from build123d import *

# Parameters (mm, degrees)
F0_W     = 294.005
F0_H     = 558.8
F1_DEPTH = 12.7
F3_D     = 4.4
F4_R     = 9.525
F6_DEPTH = 12.701


with BuildPart() as f1:
    # F0 (on Front) → F1 (new body)
    with BuildSketch(Plane.XZ):
        Rectangle(F0_W, F0_H)
    extrude(amount=F1_DEPTH)

    # F3 (through all)
    with Locations(Plane.XZ.offset(12.7)):
        with Locations((-137.4775, 269.875), (-105.7275, 269.875), (105.7275, 269.875), (137.4775, 269.875), (105.7275, -238.125), (137.4775, -238.125), (137.4775, -269.875), (105.7275, -269.875), (-105.7275, -269.875), (-137.4775, -269.875), (-137.4775, -238.125), (-105.7275, -238.125)):
            Hole(F3_D / 2)

    # F4
    f4_edges = [f1.edges().sort_by_distance(p)[0] for p in [
        (147.0025, -6.35, 279.4),
        (147.0025, -6.35, -279.4),
        (-147.0025, -6.35, -279.4),
        (-147.0025, -6.35, 279.4),
    ]]
    fillet(f4_edges, radius=F4_R)

    # F5 (on face) → F6 (cut, through all)
    with BuildSketch(Plane.XZ.offset(12.7)):
        with BuildLine():
            Line((88.9, 127), (-88.9, 127))
            ThreePointArc((-88.9, 127), (-106.8605122421, 119.5605122421), (-114.3, 101.6))
            Line((-114.3, 101.6), (-114.3, -203.2))
            ThreePointArc((-114.3, -203.2), (-106.8605122421, -221.1605122421), (-88.9, -228.6))
            Line((-88.9, -228.6), (88.9, -228.6))
            ThreePointArc((88.9, -228.6), (106.8605122421, -221.1605122421), (114.3, -203.2))
            Line((114.3, -203.2), (114.3, 101.6))
            ThreePointArc((114.3, 101.6), (106.8605122421, 119.5605122421), (88.9, 127))
        make_face()
    extrude(amount=-F6_DEPTH, mode=Mode.SUBTRACT)


solid = f1.part
Design review of the part built by this model. Coordinates are the model's own, in mm. A direction names the side the tool comes from. Give positions to 0.01 mm unless a question says otherwise; leave off trailing zeros. Order: outer loops, then holes, each group sorted by start corner. A loop starts at its lowest first (then second) coordinate and runs counter-clockwise, first axis right, second up. Notation, with made-up numbers: (71.5, 30.25) - (97.5, 30.25) arc R18 cw to (97.5, 40.25) - close; hole circle Ø5 at (-37.5, 44.25). An arc over 180 degrees is marked (long way). Use CSV: the item, a comma, the result in double quotes. Start each with the question number.
Q1. Draft analysis for pull direction Z (two halves, no side actions). For faces 1 (the face through (147.002, -6, -4)), 2 (the face through (144.14, -6.44, 276.68)), 3 (the face through (-107.06, -6.44, -220.96)), state which applies: pulls with the +Z half, pulls with the -Z half, needs draft (parallel to the pull), parting line crosses it, or undercut.
Q2. For P1, Ø7, axis at x = 105.73, z = -238.12, coming from the +Y side, flat-tipped, find the tip position at first contact; note if it passes through.
Q3. Machinability: for faces 4 (the face through (144.14, -6.44, -276.68)), 5 (the face through (107.06, -6.44, 119.36)), which of the approach directions +Z, -Z, +X, -X, +Y, -Y give a long, thin tool a straight path to every point of the face, cutting with its end or side? Answer none if there is none.
Q4. Take a section at B-B (x = -39.5). State the section outline as (y, z) points, and give its area (3 significant figures).
Q5. For line 1 (Z direction, x = -14, y = -7); line 2 (X direction, y = -7.75, z = 95); line 3 (Z direction, x = 99, y = -3.75), list the stretches that pass through material, from the lowest coordinate up.
Q6. Take a section at A-A (z = -44). State the section outline as (x, y) points, and give its area (3 significant figures).
Q7. Take a section at C-C (y = -7.25). Count the separate pieces of the cut face and the enclosed holes in it, and give its area (3 significant figures).
Calculated:
1,face 1,"needs draft"
1,face 2,"pulls with the +Z half"
1,face 3,"undercut"
2,P1,"stops at y = 0"
3,face 4,"-Z, +X, +Y, -Y"
3,face 5,"+Y, -Y"
4,outline,"(-12.7, -279.4) - (0, -279.4) - (0, -228.6) - (-12.7, -228.6) - close; (-12.7, 127) - (0, 127) - (0, 279.4) - (-12.7, 279.4) - close"
4,area,"2,580 mm²"
5,line 1,"z = -279.4 to -228.6, 127 to 279.4"
5,line 2,"x = -147 to -114.3, 114.3 to 147"
5,line 3,"z = -279.4 to -226.51, 124.91 to 279.4"
6,outline,"(-147, -12.7) - (-114.3, -12.7) - (-114.3, 0) - (-147, 0) - close; (114.3, -12.7) - (147, -12.7) - (147, 0) - (114.3, 0) - close"
6,area,"831 mm²"
7,separate pieces,"1"
7,enclosed holes,"13"
7,area,"83,300 mm²"
